Part model, mm, in its own coordinate system. A direction names the side the tool comes from. Round coordinates to 2 decimals unless told otherwise and drop trailing zeros. Loops run counter-clockwise (first coordinate to the right, second up) from the corner with the lowest first, then second, coordinate; pieces in that order, holes last. Notation, with made-up numbers: (5.25, 85) - (41.25, 85) arc R3 cw to (41.25, 90) - close; hole circle Ø2 at (44.5, -36.5). An arc over 180 degrees is marked (long way). Write each question's results on one line, items separated by ' | '. Start each with the question number.
(1) Mould opens along X. For faces 4 (the face through (-172, 100.584, -65)), 5 (the face through (-170, 0, -40)), 6 (the face through (-108.62, 22.72, -91.51)), 7 (the face through (-130, 100.584, -32)) say: released by +X, released by -X, zero draft, split by the parting line, or undercut.
(2) Drill centre lines: L1, parallel to X at y = 51, z = -48.26; L2, parallel to X at y = 79, z = -35.5; L3, parallel to Z at x = -33.02, y = 43. Where is each one in solid material? Low to high.
(3) Tool access for faces 1 (the face through (-66.04, 58, -48)), 2 (the face through (-31.213, 55.083, -29.964)), 3 (the face through (-33, 84.074, -60)): list every direction of +Z, -Z, +X, -X, +Y, -Y with a clear straight run to the whole face (end or side of a thin tool).
(4) Cut at C-C, the plane x = -112. List the corners of the cut face in (y, z), then the cut area to 3 significant figures.
(5) Cut at A-A, the plane y = 61. List the corners of the cut face in (x, z), then the cut area to 3 significant figures.
(6) Flat gauge pins, fed straight in: P1, Ø10, axis at y = 36.5, z = -22, coming from the -X side; P2, Ø5, axis at x = -102.5, z = -78, coming from the -Y side; P3, Ø4, axis at x = -63.5, z = -50, coming from the +Y side. Where does each tip first touch, or does it go through?
(7) Cut at B-B, the plane y = 22. List the corners of the cut face in (x, z), then the cut area to 3 significant figures.
from build123d import *

# Parameters (mm, degrees)
SKETCH1_W                                           = 66.04
SKETCH1_H                                           = 96.52
BOSS_EXTRUDE1_DEPTH                                 = 84.074
BOSS_EXTRUDE2_START                                 = 12.7
BOSS_EXTRUDE2_DEPTH                                 = 20.32
SKETCH1_4_R                                         = 38.1
SKETCH1_4_R_2                                       = 19.05
BOSS_EXTRUDE3_DEPTH                                 = 113.284
FILLET1_R                                           = 7.62
CSK_FOR_5_8_FLAT_HEAD_MACHINE_SCREW_100_D           = 16.66748
CSK_FOR_5_8_FLAT_HEAD_MACHINE_SCREW_100_DEPTH       = 50.8
CSK_FOR_5_8_FLAT_HEAD_MACHINE_SCREW_100_CSINK_D     = 32.3088
CSK_FOR_5_8_FLAT_HEAD_MACHINE_SCREW_100_CSINK_ANGLE = 100
CSK_FOR_5_8_FLAT_HEAD_MACHINE_SCREW_100_TIP         = 5.007416175
CUT_EXTRUDE1_DEPTH                                  = 12.7


with BuildPart() as part:
    # Sketch1 → Boss-Extrude1 (new body)
    with BuildSketch(Plane(origin=(0, 0, 0), x_dir=(1, 0, 0), z_dir=(0, 1, 0))):
        with Locations((-33.02, 48.26)):
            Rectangle(SKETCH1_W, SKETCH1_H)
    extrude(amount=BOSS_EXTRUDE1_DEPTH)

    # Sketch1_3 → Boss-Extrude2 (add)
    with BuildSketch(Plane(origin=(0, 0, 0), x_dir=(1, 0, 0), z_dir=(0, 1, 0)).offset(BOSS_EXTRUDE2_START)):
        with BuildLine():
            Line((-152.4, 10.16), (-66.04, 0))
            Line((-66.04, 0), (-66.04, 96.52))
            Line((-66.04, 96.52), (-152.4, 86.36))
            ThreePointArc((-152.4, 86.36), (-125.459231637, 75.200768363), (-114.3, 48.26))
            ThreePointArc((-114.3, 48.26), (-125.459231637, 21.319231637), (-152.4, 10.16))
        make_face()
    extrude(amount=BOSS_EXTRUDE2_DEPTH)

    # Sketch1_4 → Boss-Extrude3 (add)
    with BuildSketch(Plane(origin=(0, 0, 0), x_dir=(1, 0, 0), z_dir=(0, 1, 0))):
        with Locations((-152.4, 48.26)):
            Circle(SKETCH1_4_R)
        with Locations((-152.4, 48.26)):
            Circle(SKETCH1_4_R_2, mode=Mode.SUBTRACT)
    extrude(amount=BOSS_EXTRUDE3_DEPTH)

    # Fillet1
    fillet1_edges = [part.edges().sort_by_distance(p)[0] for p in [
        (-190.5, 113.284, -48.26),
    ]]
    fillet(fillet1_edges, radius=FILLET1_R)

    # CSK for 5_8 Flat Head Machine Screw _100
    with Locations(Plane(origin=(0, 84.074, 0), x_dir=(1, 0, 0), z_dir=(0, 1, 0))):
        with Locations((-33.02, 38.1)):
            CounterSinkHole(CSK_FOR_5_8_FLAT_HEAD_MACHINE_SCREW_100_D / 2, CSK_FOR_5_8_FLAT_HEAD_MACHINE_SCREW_100_CSINK_D / 2, depth=CSK_FOR_5_8_FLAT_HEAD_MACHINE_SCREW_100_DEPTH, counter_sink_angle=CSK_FOR_5_8_FLAT_HEAD_MACHINE_SCREW_100_CSINK_ANGLE)
            with Locations((0, 0, -(CSK_FOR_5_8_FLAT_HEAD_MACHINE_SCREW_100_DEPTH + CSK_FOR_5_8_FLAT_HEAD_MACHINE_SCREW_100_TIP / 2))):  # 118° drill point
                Cone(0, CSK_FOR_5_8_FLAT_HEAD_MACHINE_SCREW_100_D / 2, CSK_FOR_5_8_FLAT_HEAD_MACHINE_SCREW_100_TIP, mode=Mode.SUBTRACT)

    # Sketch4 → Cut-Extrude1 (cut)
    with BuildSketch(Plane(origin=(0, 113.284, 0), x_dir=(1, 0, 0), z_dir=(0, 1, 0))):
        with BuildLine():
            ThreePointArc((-165.462255431, 75.799206289), (-175.749034626, 67.852166343), (-181.789060717, 56.341677434))
            Line((-181.789060717, 56.341677434), (-171.440491942, 47.658197191))
            ThreePointArc((-171.440491942, 47.658197191), (-166.993146641, 60.505103965), (-155.113686656, 67.115726046))
            Line((-155.113686656, 67.115726046), (-165.462255431, 75.799206289))
        make_face()
        with BuildLine():
            Line((-149.686313344, 29.404273954), (-139.337744569, 20.720793711))
            ThreePointArc((-139.337744569, 20.720793711), (-129.050965374, 28.667833657), (-123.010939283, 40.178322566))
            Line((-123.010939283, 40.178322566), (-133.359508058, 48.861802809))
            ThreePointArc((-133.359508058, 48.861802809), (-133.352377163, 48.560938957), (-133.35, 48.26))
            ThreePointArc((-133.35, 48.26), (-138.002114204, 35.78589143), (-149.686313344, 29.404273954))
        make_face()
        with BuildLine():
            ThreePointArc((-123.010939283, 40.178322566), (-129.050965374, 28.667833657), (-139.337744569, 20.720793711))
            Line((-139.337744569, 20.720793711), (-103.383523075, -9.448380284))
            Line((-103.383523075, -9.448380284), (-87.056717789, 10.009148571))
            Line((-87.056717789, 10.009148571), (-123.010939283, 40.178322566))
        make_face()
        with BuildLine():
            Line((-181.640283335, 89.374183536), (-197.967088621, 69.916654681))
            Line((-197.967088621, 69.916654681), (-181.789060717, 56.341677434))
            ThreePointArc((-181.789060717, 56.341677434), (-175.749034626, 67.852166343), (-165.462255431, 75.799206289))
            Line((-165.462255431, 75.799206289), (-181.640283335, 89.374183536))
        make_face()
    extrude(amount=-CUT_EXTRUDE1_DEPTH, mode=Mode.SUBTRACT)


solid = part.part
A:
1) face 4: undercut | face 5: zero draft | face 6: released by -X | face 7: undercut
2) L1: -190.5 to -171.45, -133.35 to -114.3, -66.04 to 0 | L2: -188.3 to -166.55, -138.25 to -116.5, -66.04 to -42.79, -23.25 to 0 | L3: -96.52 to -46.43, -29.77 to 0
3) face 1: +Z, -Z, +Y | face 2: +Y | face 3: +Z, -Z, +X, +Y
4) outline: (12.7, -91.11) - (33.02, -91.11) - (33.02, -5.41) - (12.7, -5.41) - close | area: 1,740 mm2
5) outline: circle Ø76.2 at (-152.4, -48.26); (-66.04, -96.52) - (0, -96.52) - (0, 0) - (-66.04, 0) - close; hole circle Ø38.1 at (-152.4, -48.26); hole circle Ø16.67 at (-33.02, -38.1) | area: 9,580 mm2
6) P1: x = -184.02 | P2: y = 12.7 | P3: y = 84.07
7) outline: (-152.4, -86.36) - (-66.04, -96.52) - (0, -96.52) - (0, 0) - (-66.04, 0) - (-152.4, -10.16) arc R38.1 ccw to start; hole circle Ø38.1 at (-152.4, -48.26) | area: 15,000 mm2
